from build123d import *

# Parameters (mm, degrees)
F0_R     = 3.5
F1_DEPTH = 8
F3_DEPTH = 3
F4_R     = 2.5
F5_DEPTH = 25
F6_SIZE  = 0.99999


# Not quite as in the source:
# - a fillet or chamfer is up to 0.001 mm smaller than in the source, because OpenCascade refuses the exact size


with BuildPart() as f1:
    # F0 (on Front) → F1 (new body)
    with BuildSketch(Plane.XZ):
        Circle(F0_R)
    extrude(amount=F1_DEPTH)

    # F2 (on face) → F3 (cut)
    with BuildSketch(Plane.XZ.offset(8)):
        Polygon((2.5, 1.443375673), (0, 2.8867513459), (-2.5, 1.443375673), (-2.5, -1.443375673), (0, -2.8867513459), (2.5, -1.443375673), align=None)
    extrude(amount=-F3_DEPTH, mode=Mode.SUBTRACT)

    # F4 (on face) → F5 (cut)
    with BuildSketch(Plane.XZ.offset(5)):
        Circle(F4_R)
    extrude(amount=-F5_DEPTH, mode=Mode.SUBTRACT)

    # F6 (size 1 in the source; OpenCascade refuses exactly that, so slightly less here)
    f6_edges = [f1.edges().sort_by_distance(p)[0] for p in [
        (-3.5, 0, 0),
    ]]
    chamfer(f6_edges, length=F6_SIZE)


solid = f1.part
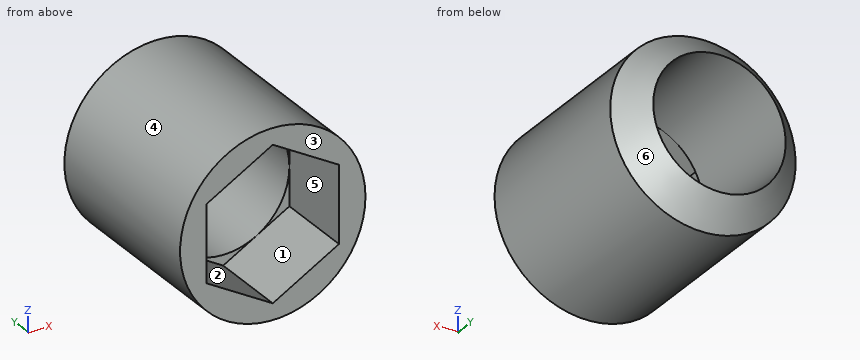
Build history of the part. All positions in model axes, mm. Face numbers are marked on the shaded views. A direction names the side the tool comes from. Round coordinates to 2 decimals unless told otherwise and drop trailing zeros. Order: outer loops, then holes, each group sorted by start corner. A loop starts at its lowest first (then second) coordinate and runs counter-clockwise, first axis right, second up. Notation, with made-up numbers: M 71.5,36.5 L 112.5,36.5 A19 ccw 112.5,51.5 Z; hole C 4.5,12 d11. An arc over 180 degrees is marked long. Use CSV: the item, a comma, the result in double quotes. Start each with the question number.
(1) Flat gauge pins, fed straight in: P1, Ø0.6, axis at x = -2, z = -1, coming from the -Y side; P2, Ø1.5, axis at y = -3, z = -1.5, coming from the -X side; P3, Ø3, axis at y = -1.5, z = -3, coming from the +X side. Where does each tip first touch, or does it go through?
(2) Tool access for the marked faces 5 and 6: list every direction of +Z, -Z, +X, -X, +Y, -Y with a clear straight run to the whole face (end or side of a thin tool).
(3) Drill centre lines: probe 1 along Z at (x, y) = (0, -3.3); probe 2 along X at (y, z) = (-1.75, 1.25); probe 3 along X at (y, z) = (-2.75, -2.25). Where is each one in solid material? Low to high.
(4) Cut at A-A on y = -6.5. List the corners of the cut face in (x, z), then the cut area to 3 significant figures.
(5) Cut at B-B on y = -3. List the corners of the cut face in (x, z), then the cut area to 3 significant figures.
(6) Mould opens along X. For the marked faces 1, 2, 3 and 4 say: +X half, -X half, draft (parallel to the pull), parting line (faces both ways), or undercut.
Findings:
1,P1,"stops at y = -5"
1,P2,"stops at x = -3.42"
1,P3,"stops at x = 3.16"
2,face 5,"-Y"
2,face 6,"+Y"
3,probe 1,"z = -3.5 to -2.5, 2.5 to 3.5"
3,probe 2,"x = -3.27 to -2.17, 2.17 to 3.27"
3,probe 3,"x = -2.68 to -1.09, 1.09 to 2.68"
4,outline,"C 0,0 d7; hole M -2.5,-1.44 L 0,-2.89 L 2.5,-1.44 L 2.5,1.44 L 0,2.89 L -2.5,1.44 Z"
4,area,"16.8 mm^2"
5,outline,"C 0,0 d7; hole C 0,0 d5"
5,area,"18.8 mm^2"
6,face 1,"undercut"
6,face 2,"undercut"
6,face 3,"draft"
6,face 4,"parting line"
